The model under review builds one solid part; all positions refer to its coordinate system, in mm. A direction names the side the tool comes from. Round coordinates to 2 decimals unless told otherwise and drop trailing zeros. Write each loop counter-clockwise with the first axis right and the second up, starting at its lowest first coordinate (ties: lowest second). Pieces come first, ordered by that corner, then holes. Notation, with made-up numbers: (-21, 17.5) - (-4, 17.5) arc R13 cw to (-4, 25.5) - close; hole circle Ø4 at (65, 15.25). An arc over 180 degrees is marked (long way). Write each question's results on one line, items separated by ' | '.
Autodesk Inventor part; units mm, degrees
ref_plane "Work Plane1" through (0, 0, 0) normal (-0.5, -0.866, 0) x (0, 0, 1)
ref_plane "YZ Plane" through (0, 0, 0) normal (1, 0, 0) x (0, 1, 0)
ref_plane "XY Plane" through (0, 0, 0) normal (0, 0, 1) x (1, 0, 0)
sketch "Sketch1" plane through (0, 0, 0) normal (0, 0, 1) x (1, 0, 0)
  circle A0 centre (0, 0) radius 15
  circle A1 centre (0, 0) radius 4
  point P0 (12, 0)
  point P1 (-6, 10.3923)
  point P2 (-6, -10.3923)
  dimension "d0" = 30
  dimension "d1" = 12
  dimension "d2" = 8
  dimension "d5" = 360
extrude "Plate1" add sketch "Sketch1" along normal blind 10
hole "Hole1" at (12, 0, 0) at (-6, 10.3923, 0) at (-6, -10.3923, 0) direction (0, 0, 1) diameter 3.242 depth 15 tip angle 118
sketch "Sketch2" plane through (0, 0, 0) normal (1, 0, 0) x (0, 1, 0)
  line L0 (4, 0) -> (-4, 0)
  point P0 (0, 0)
  point P1 (0, 5)
  dimension "d15" = 5
hole "Hole2" at (0, 0, 5) direction (-1, 0, 0) diameter 2.459 end through all
ref_plane "Work Plane1" through (0, 0, 0) normal (-0.5, -0.866, 0) x (0, 0, 1)
sketch "Sketch3" plane through (0, 0, 0) normal (-0.5, -0.866, 0) x (0, 0, 1)
  point P0 (0, 0)
  point P1 (5, 3.9111)
  point P2 (5, 0)
  dimension "d24" = 5
hole "Hole3" at (0, 0, 5) direction (0.5, 0.866, 0) diameter 2.459 end through all
equation "\"d7\" = Thickness"
equation "\"BendReliefDepth\" = 0.5 * Thickness"
properties part number "asmountAs4" material "Aluminum 6061"
Q1. We need section D-D (y = -11). State the section outline as (x, z) points.
Evaluation:
outline: (-10.2, 0) - (-7.5, 0) - (-7.5, 10) - (-10.2, 10) - close; (-4.5, 0) - (10.2, 0) - (10.2, 10) - (-4.5, 10) - close
Q2. Tool access review of faces 1 (the cylindrical face through (-4.418, -10.744, 5.07)), 2 (the cylindrical face through (-9.48, -0.05, 6.23)): name each direction out of +Z, -Z, +X, -X, +Y, -Y from which nothing blocks a thin tool from reaching the whole face with its end or side.
Evaluation:
face 1: +Z, -Z | face 2: -X
Q3. Insertion check: P1, Ø7, axis at x = 0, y = 0, coming from the -Z side; P2, Ø1, axis at y = 10.5, z = 5, coming from the +X side; P3, Ø1.5, axis at y = -3, z = 4, coming from the -X side; P4, Ø4, axis at y = 4, z = 1.5, coming from the -X side. Each pin has a flat end and moves straight along its axis. Give the tip position at first contact, or say it passes through.
Evaluation:
P1: passes through | P2: stops at x = 11.18 | P3: stops at x = -14.83 | P4: stops at x = -14.87
Q4. We need section B-B (y = 0). State the section outline as (x, z) points, plus the area to 3 significant figures.
Evaluation:
outline: (-15, 0) - (-4, 0) - (-4, 3.77) - (-15, 3.77) - close; (-15, 6.23) - (-4, 6.23) - (-4, 10) - (-15, 10) - close; (4, 0) - (10.38, 0) - (10.38, 10) - (4, 10) - close; (13.62, 0) - (15, 0) - (15, 10) - (13.62, 10) - close | area: 161 mm^2
Q5. We need section A-A (x = 0). State the section outline as (y, z) points.
Evaluation:
outline: (-15, 0) - (-4, 0) - (-4, 10) - (-15, 10) - close; (4, 0) - (15, 0) - (15, 10) - (4, 10) - close
Q6. We need section C-C (z = 4.75). State the section outline as (x, y) points.
Evaluation:
outline: (-14.95, -1.2) arc R15 ccw (long way) to (8.52, 12.35) - (2.95, 2.7) arc R4 cw (long way) to (-3.81, -1.2) - close; (-14.95, 1.2) - (-3.81, 1.2) arc R4 cw to (0.86, 3.91) - (6.43, 13.55) arc R15 ccw to start; hole circle Ø3.24 at (-6, -10.39); hole circle Ø3.24 at (-6, 10.39); hole circle Ø3.24 at (12, 0)
Q7. The part is to be moulded in two halves that separate along Z. For faces 3 (the flat face through (3, -3, 0)), 4 (the cylindrical face through (10.393, -0.211, 5.07)), 5 (the cylindrical face through (5.149, 7.976, 3.864)), say which applies: released by +Z, released by -Z, zero draft, split by the parting line, or undercut.
Evaluation:
face 3: released by -Z | face 4: zero draft | face 5: undercut
Q8. For probe 1 along Y at (x, z) = (0, 3); probe 2 along Y at (x, z) = (-6, 6); probe 3 along Y at (x, z) = (-6, 6.75), list the stretches that pass through material, from the lowest coordinate up.
Evaluation:
probe 1: y = -15 to -4, 4 to 15 | probe 2: y = -13.75 to -12.01, -8.77 to -0.72, 0.72 to 8.77, 12.01 to 13.75 | probe 3: y = -13.75 to -12.01, -8.77 to 8.77, 12.01 to 13.75
